For this review, take the finished solid that the model builds, in its own axes (mm). A direction names the side the tool comes from. Round coordinates to 2 decimals unless told otherwise and drop trailing zeros. Loops run counter-clockwise (first coordinate to the right, second up) from the corner with the lowest first, then second, coordinate; pieces in that order, holes last.
```python
from build123d import *

# Parameters (mm, degrees)
BOSS_EXTRU_1_DEPTH      = 0.5
BOSS_EXTRU_2_DEPTH      = 3
ESQUISSE1_4_R           = 0.4
ENL_V_MAT_EXTRU_1_DEPTH = 1.5
BOSS_EXTRU_3_DEPTH      = 3
BOSS_EXTRU_3_DEPTH_BACK = 0.5


with BuildPart() as part:
    # Esquisse1 → Boss.-Extru.1 (new body)
    with BuildSketch(Plane.XY):
        with BuildLine():
            Line((-3.31662479, 5), (3.31662479, 5))
            ThreePointArc((3.31662479, 5), (6, 0), (3.31662479, -5))
            Line((3.31662479, -5), (-3.31662479, -5))
            ThreePointArc((-3.31662479, -5), (-6, 0), (-3.31662479, 5))
        make_face()
    extrude(amount=-BOSS_EXTRU_1_DEPTH)

    # Esquisse1_3 → Boss.-Extru.2 (add)
    with BuildSketch(Plane.XY):
        with BuildLine():
            Line((3.31662479, 5), (-3.31662479, 5))
            ThreePointArc((-3.31662479, 5), (-6, 0), (-3.31662479, -5))
            Line((-3.31662479, -5), (-2.5, -5))
            Line((-2.5, -5), (2.5, -5))
            Line((2.5, -5), (3.31662479, -5))
            ThreePointArc((3.31662479, -5), (6, 0), (3.31662479, 5))
        make_face()
        with BuildLine():
            ThreePointArc((-3, -4), (-5, 0), (-3, 4))
            Line((-3, 4), (3, 4))
            ThreePointArc((3, 4), (5, 0), (3, -4))
            Line((3, -4), (-3, -4))
        make_face(mode=Mode.SUBTRACT)
    extrude(amount=BOSS_EXTRU_2_DEPTH)

    # Esquisse1_4 → Enl_v. mat.-Extru.1 (cut, through all)
    with BuildSketch(Plane.XY):
        with Locations((-3, 0)):
            Circle(ESQUISSE1_4_R)
        with Locations((3, 0)):
            Circle(ESQUISSE1_4_R)
    extrude(amount=-ENL_V_MAT_EXTRU_1_DEPTH, mode=Mode.SUBTRACT)

    # Esquisse1_5 → Boss.-Extru.3 (add, two sides)
    with BuildSketch(Plane.XY) as boss_extru_3_sk:
        Polygon((2.5, -5), (-2.5, -5), (-2.5, -9), (-4, -9), (-4, -12), (4, -12), (4, -9), (2.5, -9), align=None)
    extrude(amount=BOSS_EXTRU_3_DEPTH)
    extrude(boss_extru_3_sk.sketch, amount=-BOSS_EXTRU_3_DEPTH_BACK)


solid = part.part
```
(1) Add section D-D (y = 3.75). Give the boundary of the cut face in (x, z).
(2) Add section B-B (z = 2.5). Give the boundary of the cut face in (x, y), plus the area to 3 significant figures.
(3) Add section A-A (y = 0). Give the boundary of the cut face in (x, z), plus the area to 3 significant figures.
(4) For L1, parallel to Y at x = 3, z = -0.3; L2, parallel to Y at x = -0.5, z = 0.9; L3, parallel to Y at x = -3.75, z = 2.55, list the stretches that pass through material, from the lowest coordinate up.
(5) For faces 4 (the flat face through (3, -5, 1)), 5 (the flat face through (0, -4, 1)), 6 (the flat face through (-3, -5, 1)), list the 3-axis set-ups (+Z, -Z, +X, -X, +Y, -Y) from which the entire face can be reached by the end or side of a thin tool; tool diameter is ignored.
(6) Insertion check: pin 1 Ø1.5 at (y, z) = (-10, 2) entering from +X. The pin has a flat end and moves straight along its axis. Give the tip position at first contact, or say it passes through.
(7) The part is to be moulded in two halves that separate along Y. For faces 1 (the flat face through (0, -12, 1)), 2 (the flat face through (2.5, -7, 1)), 3 (the flat face through (0, -1, -0.5)), say which applies: pulls with the +Y half, pulls with the -Y half, needs draft (parallel to the pull), parting line crosses it, or undercut.
(8) Add section C-C (x = 0.75). Give the boundary of the cut face in (y, z), plus the area to 3 significant figures.
Outcome:
1. outline: (-4.68, -0.5) - (4.68, -0.5) - (4.68, 3) - (3.31, 3) - (3.31, 0) - (-3.31, 0) - (-3.31, 3) - (-4.68, 3) - close
2. outline: (-4, -12) - (4, -12) - (4, -9) - (2.5, -9) - (2.5, -5) - (3.32, -5) arc R6 ccw to (3.32, 5) - (-3.32, 5) arc R6 ccw to (-3.32, -5) - (-2.5, -5) - (-2.5, -9) - (-4, -9) - close; hole (-3, -4) - (3, -4) arc R5 ccw to (3, 4) - (-3, 4) arc R5 ccw to start
2. area: 77.7 mm2
3. outline: (-6, -0.5) - (-3.4, -0.5) - (-3.4, 0) - (-5, 0) - (-5, 3) - (-6, 3) - close; (-2.6, -0.5) - (2.6, -0.5) - (2.6, 0) - (-2.6, 0) - close; (3.4, -0.5) - (6, -0.5) - (6, 3) - (5, 3) - (5, 0) - (3.4, 0) - close
3. area: 11.2 mm2
4. L1: y = -12 to -9, -5 to -0.4, 0.4 to 5
4. L2: y = -12 to -4, 4 to 5
4. L3: y = -12 to -9, -4.68 to -3.31, 3.31 to 4.68
5. face 4: +Z, -Z, +X
5. face 5: +Z
5. face 6: +Z, -Z, -X
6. pin 1: stops at x = 4
7. face 1: pulls with the -Y half
7. face 2: undercut
7. face 3: needs draft
8. outline: (-12, -0.5) - (5, -0.5) - (5, 3) - (4, 3) - (4, 0) - (-4, 0) - (-4, 3) - (-12, 3) - close
8. area: 35.5 mm2
